from build123d import *

# Parameters (mm, degrees)
PAD_DEPTH       = 5
POCKET_DEPTH    = 4
SKETCH001_W     = 30
SKETCH001_H     = 28
PAD001_DEPTH    = 5
SKETCH003_W     = 29
SKETCH003_H     = 27
POCKET001_DEPTH = 5
SKETCH004_W     = 2
SKETCH004_H     = 2
POCKET002_DEPTH = 4
FILLET_R        = 1
FILLET001_R     = 1
FILLET002_R     = 1
FILLET003_R     = 0.5


with BuildPart() as part:
    # Sketch → Pad (new body)
    with BuildSketch(Plane.XY):
        Polygon((36.5, 7.5), (19.5, 7.5), (19.5, 18.5), (-19.5, 18.5), (-19.5, -18.5), (19.5, -18.5), (19.5, -7.5), (36.5, -7.5), align=None)
    extrude(amount=PAD_DEPTH)

    # Sketch002 → Pocket (cut)
    with BuildSketch(Plane.XY.offset(1)):
        Polygon((35.5, 6.5), (18.5, 6.5), (18.5, 17.5), (-18.5, 17.5), (-18.5, -17.5), (18.5, -17.5), (18.5, -6.5), (35.5, -6.5), align=None)
    extrude(amount=POCKET_DEPTH, mode=Mode.SUBTRACT)

    # Sketch001 → Pad001 (join)
    with BuildSketch(Plane.XY):
        Rectangle(SKETCH001_W, SKETCH001_H)
    extrude(amount=PAD001_DEPTH)

    # Sketch003 → Pocket001 (cut)
    with BuildSketch(Plane.XY):
        Rectangle(SKETCH003_W, SKETCH003_H)
    extrude(amount=POCKET001_DEPTH, mode=Mode.SUBTRACT)

    # Sketch004 → Pocket002 (cut)
    with BuildSketch(Plane.XY.offset(1)):
        with Locations((35.5, 0)):
            Rectangle(SKETCH004_W, SKETCH004_H)
    extrude(amount=POCKET002_DEPTH, mode=Mode.SUBTRACT)

    # Fillet
    fillet_edges = [part.edges().sort_by_distance(p)[0] for p in [
        (-15, -14, 3),
        (15, -14, 3),
        (15, 14, 3),
        (-15, 14, 3),
    ]]
    fillet(fillet_edges, radius=FILLET_R)

    # Fillet001
    fillet001_edges = [part.edges().sort_by_distance(p)[0] for p in [
        (18.5, 6.5, 3),
        (18.5, -6.5, 3),
    ]]
    fillet(fillet001_edges, radius=FILLET001_R)

    # Fillet002
    fillet002_edges = [part.edges().sort_by_distance(p)[0] for p in [
        (-19.5, 18.5, 2.5),
        (-19.5, -18.5, 2.5),
        (19.5, 18.5, 2.5),
        (36.5, 7.5, 2.5),
        (36.5, -7.5, 2.5),
        (19.5, -18.5, 2.5),
    ]]
    fillet(fillet002_edges, radius=FILLET002_R)

    # Fillet003
    fillet003_edges = [part.edges().sort_by_distance(p)[0] for p in [
        (35.5, -1, 3),
        (35.5, 1, 3),
    ]]
    fillet(fillet003_edges, radius=FILLET003_R)


solid = part.part
Work out the finished part from the listing and answer in its coordinate system (mm). A direction names the side the tool comes from. Round coordinates to 2 decimals unless told otherwise and drop trailing zeros. Order: outer loops, then holes, each group sorted by start corner. A loop starts at its lowest first (then second) coordinate and runs counter-clockwise, first axis right, second up. Notation, with made-up numbers: M -7,-9.75 L 11,-9.75 A11 ccw 11,-4.75 Z; hole C -23,-39 d4. An arc over 180 degrees is marked long. One line per item, written item: value.
Q1. Straight lines are drawn through the part: line 1 (Y direction, x = 0, z = 2.05); line 2 (X direction, y = 4.5, z = 1.45); line 3 (X direction, y = 10.5, z = 4.35). For each, find the intervals that lie inside material, in ascending order.
Derived:
line 1: -18.5 to -17.5, -14 to -13.5, 13.5 to 14, 17.5 to 18.5
line 2: -19.5 to -18.5, -15 to -14.5, 14.5 to 15, 35.5 to 36.5
line 3: -19.5 to -18.5, -15 to -14.5, 14.5 to 15, 18.5 to 19.5
Q2. For faces 1 (the face through (-14.5, 0, 2)), 2 (the face through (19.5, 12, 2)), 3 (the face through (0, -14, 3)), 4 (the face through (19.5, -13, 2)), determine the directions among +Z, -Z, +X, -X, +Y, -Y from which every point of the face is accessible in a straight line to the end or side of a thin tool.
Derived:
face 1: +Z, -Z
face 2: +Z, -Z, +X, +Y
face 3: +Z
face 4: +Z, -Z, +X, -Y
Q3. Flat-ended cylindrical pins translate along their axes: pin 1 (2 mm diameter, centred on x = 27, z = 0.5, fed in from +Y); pin 2 (1 mm diameter, centred on x = 29.5, z = 1, fed in from -Y); pin 3 (3 mm diameter, centred on x = 20.5, z = 4.5, fed in from +Y); pin 4 (10.5 mm diameter, centred on x = -1, y = 5, fed in from +Z). Find the tip coordinate at first contact, or state that the pin passes through.
Derived:
pin 1: y = 7.5
pin 2: y = -7.5
pin 3: y = 18.37
pin 4: through
Q4. Find section D-D on x = 30. Write down the section's boundary in (y, z), then the cut area to 3 significant figures.
Derived:
outline: M -7.5,0 L 7.5,0 L 7.5,5 L 6.5,5 L 6.5,1 L -6.5,1 L -6.5,5 L -7.5,5 Z
area: 23.0 mm²
Q5. Determine the mould class of faces 5 (the face through (28, 7.5, 2)), 6 (the face through (27, -6.5, 3)), 7 (the face through (0, -18.5, 2)), 8 (the face through (-19.5, 0, 2)) for opening direction Y: released by +Y, released by -Y, zero draft, split by the parting line, or undercut.
Derived:
face 5: released by +Y
face 6: undercut
face 7: released by -Y
face 8: zero draft
Q6. Find section C-C on z = 2.55. Give the number of separate pieces and of enclosed holes in the cut face, then the cut area to 3 significant figures.
Derived:
separate pieces: 2
enclosed holes: 1
area: 234 mm²
Q7. Find section B-B on x = -13. Write down the section's boundary in (y, z).
Derived:
outline: M -18.5,0 L -13.5,0 L -13.5,5 L -14,5 L -14,1 L -17.5,1 L -17.5,5 L -18.5,5 Z; M 13.5,0 L 18.5,0 L 18.5,5 L 17.5,5 L 17.5,1 L 14,1 L 14,5 L 13.5,5 Z
Q8. Find section A-A on y = 9. Write down the section's boundary in (x, z).
Derived:
outline: M -19.5,0 L -14.5,0 L -14.5,5 L -15,5 L -15,1 L -18.5,1 L -18.5,5 L -19.5,5 Z; M 14.5,0 L 19.5,0 L 19.5,5 L 18.5,5 L 18.5,1 L 15,1 L 15,5 L 14.5,5 Z
